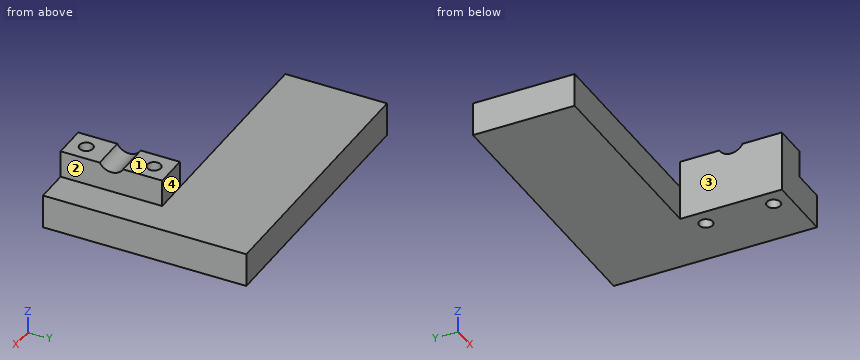
from build123d import *

# Parameters (mm, degrees)
PAD005_DEPTH    = 10
SKETCH009_W     = 10
SKETCH009_H     = 30
PAD006_DEPTH    = 8
SKETCH010_R     = 4
POCKET003_DEPTH = 10
SKETCH011_R     = 2
POCKET004_DEPTH = 20
SKETCH012_R     = 2
POCKET005_DEPTH = 20


with BuildPart() as part:
    # Sketch008 → Pad005 (new body)
    with BuildSketch(Plane(origin=(0, 0, 0), x_dir=(1, 0, 0), z_dir=(0, 0, -1))):
        Polygon((280, 160), (220, 160), (220, 130), (300, 130), (300, 190), (280, 190), align=None)
    extrude(amount=PAD005_DEPTH)

    # Sketch009 → Pad006 (new body)
    with BuildSketch(Plane.XY):
        with Locations((285, -175)):
            Rectangle(SKETCH009_W, SKETCH009_H)
    extrude(amount=PAD006_DEPTH)

    # Sketch010 → Pocket003 (cut)
    with BuildSketch(Plane(origin=(280, 0, 0), x_dir=(0, -1, 0), z_dir=(-1, 0, 0))):
        with Locations((175, 10)):
            Circle(SKETCH010_R)
    extrude(amount=-POCKET003_DEPTH, mode=Mode.SUBTRACT)

    # Sketch011 → Pocket004 (cut)
    with BuildSketch(Plane.XY.offset(8)):
        with Locations((285, -185)):
            Circle(SKETCH011_R)
    extrude(amount=-POCKET004_DEPTH, mode=Mode.SUBTRACT)

    # Sketch012 → Pocket005 (cut)
    with BuildSketch(Plane.XY.offset(8)):
        with Locations((285, -165)):
            Circle(SKETCH012_R)
    extrude(amount=-POCKET005_DEPTH, mode=Mode.SUBTRACT)


solid = part.part
The model under review builds one solid part; all positions refer to its coordinate system, in mm. Face numbers are marked on the shaded views. A direction names the side the tool comes from. Coordinates: 2 decimals unless noted, no trailing zeros. Write each loop counter-clockwise with the first axis right and the second up, starting at its lowest first coordinate (ties: lowest second). Pieces come first, ordered by that corner, then holes. Notation, with made-up numbers: (14, 74) - (73, 74) arc R21 ccw to (73, 107) - close; hole circle Ø4 at (57, 41). An arc over 180 degrees is marked (long way). Answer as a JSON object with one key per item and string values. Group by question number.
1. Add section B-B (x = 285). Give the boundary of the cut face in (y, z), plus the area to 3 significant figures.
2. Add section A-A (z = -5). Give the boundary of the cut face in (x, y), plus the area to 3 significant figures.
3. To check wall thickness, follow probe 1 along Y at (x, z) = (285, -3.75); probe 2 along Y at (x, z) = (285, 1.75); probe 3 along X at (y, z) = (-165, 0.25). State the ranges of each line that lie inside material, in increasing order.
4. Add section C-C (y = -165). Give the boundary of the cut face in (x, z), plus the area to 3 significant figures.
5. Add section D-D (x = 227). Give the boundary of the cut face in (y, z).
6. Clearance check with flat-ended pins moving along their axes: pin 1 Ø2.5 at (y, z) = (-175, 3.5) entering from +X; pin 2 Ø3 at (x, z) = (239.5, -7) entering from -Y; pin 3 Ø4 at (x, y) = (265.5, -148.5) entering from +Z; pin 4 Ø4.5 at (x, y) = (285, -165) entering from +Z. State where each tip first meets the part, or that it passes through.
7. Machinability: for the marked faces 1, 2, 3 and 4, which of the approach directions +Z, -Z, +X, -X, +Y, -Y give a long, thin tool a straight path to every point of the face, cutting with its end or side? Answer none if there is none.
Findings:
{
 "1": {"outline": "(-190, -10) - (-187, -10) - (-187, 8) - (-190, 8) - close; (-183, -10) - (-167, -10) - (-167, 8) - (-171.54, 8) arc R4 cw to (-178.46, 8) - (-183, 8) - close; (-163, -10) - (-130, -10) - (-130, 0) - (-160, 0) - (-160, 8) - (-163, 8) - close", "area": "686 mm²"},
 "2": {"outline": "(220, -160) - (280, -160) - (280, -190) - (300, -190) - (300, -130) - (220, -130) - close; hole circle Ø4 at (285, -185); hole circle Ø4 at (285, -165)", "area": "2,970 mm²"},
 "3": {"probe 1": "-190 to -187, -183 to -167, -163 to -130", "probe 2": "-190 to -187, -183 to -167, -163 to -160", "probe 3": "280 to 283, 287 to 290"},
 "4": {"outline": "(280, -10) - (283, -10) - (283, 8) - (280, 8) - close; (287, -10) - (300, -10) - (300, 0) - (290, 0) - (290, 8) - (287, 8) - close", "area": "208 mm²"},
 "5": {"outline": "(-160, -10) - (-130, -10) - (-130, 0) - (-160, 0) - close"},
 "6": {"pin 1": "x = 290", "pin 2": "y = -160", "pin 3": "z = 0", "pin 4": "z = 8"},
 "7": {"face 1": "+Z, +X, -X, +Y, -Y", "face 2": "+Z, +X, +Y, -Y", "face 3": "+Z, -Z, -X, -Y", "face 4": "+Z, +X, -X, +Y"}
}
